Source: CAD feature listing. Evaluate the final solid. Frame: model axes, mm. A direction names the side the tool comes from. Coordinates: 2 decimals unless noted, no trailing zeros. Order: outer loops, then holes, each group sorted by start corner. A loop starts at its lowest first (then second) coordinate and runs counter-clockwise, first axis right, second up.
Item 1: Section A-A on x = 9. Return the cut outline in (y, z).
Item 2: Contact query for flat-ended pins moving along their axis: P1, Ø7.5, axis at x = -8, y = -24, coming from the -Z side; P2, Ø12, axis at y = -14.5, z = 5.5, coming from the +X side; P3, Ø1, axis at x = 31, z = 12, coming from the +Y side; P4, Ø5, axis at x = 9, y = -7, coming from the -Z side. Output: stop coordinate, or through.
Item 3: Section C-C on y = 3. Return the cut outline in (x, z), then the cut area to 3 significant figures.
Item 4: Section D-D on z = 13.5. Return the cut outline in (x, y), then the cut area to 3 significant figures.
Item 5: Section B-B on z = 2.25. Return the cut outline in (x, y), then the cut area to 3 significant figures.
Item 6: Mould query, pull axis Y, two halves, no side actions, for faces 1 (the cylindrical face through (8.404, -9.685, 9.86)), 2 (the flat face through (0, 8, 10)), 3 (the flat face through (-7.804, 7.534, 9.86)), 4 (the cylindrical face through (-2.038, -28.315, 14.93)). Classes: released by +Y, released by -Y, zero draft, split by the parting line, or undercut.
Item 7: Ray query, line 1 (Y direction, x = 9, z = 4.5); line 2 (X direction, y = 5.5, z = 1.25); line 3 (X direction, y = 6, z = 16.5). Return the intervals inside material, ascending.
Item 8: Reachability of faces 5 (the flat face through (32.644, -13.92, 9.86)), 6 (the flat face through (24, 13.085, 10)), 7 (the flat face through (17.5, 7, 10)) from +Z, -Z, +X, -X, +Y, -Y: full face, straight path, thin tool, end or side. Return the list, or none.
from build123d import *
from OCP.BRepFilletAPI import BRepFilletAPI_MakeChamfer

# Parameters (mm, degrees)
SKETCH_1_R          = 2.75
EXTRUDE_1_DEPTH     = 20
CHAMFER_1_SIZE      = 1
CHAMFER_1_SIZE2     = 1.414213562
FILLET_1_R          = 2.5
SKETCH_2_W          = 28.23976686
SKETCH_2_H          = 12.215936495
CUT_EXTRUDE_1_DEPTH = 57.915812899
EXTRUDE_START       = -10
EXTRUDE_2_DEPTH     = 10
SKETCH_4_R          = 1.65
CUT_EXTRUDE_2_DEPTH = 10


with BuildPart() as part:
    # 草图1 → 凸台-拉伸1 (new body)
    with BuildSketch(Plane.XY):
        with BuildLine():
            Line((0, 0), (0, 18))
            Line((0, 18), (-5, 18))
            Line((-5, 18), (-10.312177826, -1.825317547))
            ThreePointArc((-10.312177826, -1.825317547), (-2.044709461, -23.66589163), (21.291049633, -22.769199403))
            Line((21.291049633, -22.769199403), (44.319805153, -4.819805153))
            Line((44.319805153, -4.819805153), (49.319805153, -4.819805153))
            Line((49.319805153, -4.819805153), (17.5, 27))
            Line((17.5, 27), (17.5, 0))
            Line((17.5, 0), (0, 0))
        make_face()
        with Locations((9, -7)):
            Circle(SKETCH_1_R, mode=Mode.SUBTRACT)
    extrude(amount=EXTRUDE_1_DEPTH)

    # 倒角1: one chamfer whose edges measure the first distance from different faces: ONE call of the kernel's chamfer builder (chamfer() names one face for all edges)
    chamfer_1_edges_1 = [part.edges().sort_by_distance(p)[0] for p in [
        (-5, 18, 10),
    ]]
    chamfer_1_side_1 = [part.faces().sort_by_distance(p)[0] for p in [
        (-2.5, 18, 10),
    ]]
    chamfer_1_edges_2 = [part.edges().sort_by_distance(p)[0] for p in [
        (0, 18, 10),
    ]]
    chamfer_1 = BRepFilletAPI_MakeChamfer(part.part.solid().wrapped)
    for e in chamfer_1_edges_1:
        chamfer_1.Add(CHAMFER_1_SIZE, CHAMFER_1_SIZE2, e.wrapped, chamfer_1_side_1[0].wrapped)  # the first distance lies on this face
    for e in chamfer_1_edges_2:
        chamfer_1.Add(CHAMFER_1_SIZE, e.wrapped)
    add(Compound.cast(chamfer_1.Shape()), mode=Mode.REPLACE)

    # 圆角1
    # the kernel refuses this fillet: 2.5 mm, written as the material it takes off along each edge
    with BuildSketch(Plane(origin=(17.5, 27, -15.088834765), x_dir=(0, -1, 0), z_dir=(0, 0, 1))) as fillet_1_piece_1:
        with BuildLine():
            CenterArc((FILLET_1_R * 2.41421356237, FILLET_1_R), FILLET_1_R, 135, 135)
            Line((FILLET_1_R * 1.70710678119, FILLET_1_R * 1.70710678119), (FILLET_1_R * 1.69296464556, FILLET_1_R * 1.72124891681))
            Line((FILLET_1_R * 1.69296464556, FILLET_1_R * 1.72124891681), (-FILLET_1_R * 0.0141421356237, FILLET_1_R * 0.0141421356237))
            Line((-FILLET_1_R * 0.0141421356237, FILLET_1_R * 0.0141421356237), (0, -FILLET_1_R * 0.02))
            Line((0, -FILLET_1_R * 0.02), (FILLET_1_R * 2.41421356237, -FILLET_1_R * 0.02))
            Line((FILLET_1_R * 2.41421356237, -FILLET_1_R * 0.02), (FILLET_1_R * 2.41421356237, 0))
        make_face()
    extrude(amount=50.17766953, mode=Mode.SUBTRACT)
    with BuildSketch(Plane(origin=(49.319805153, -4.819805153, -14.527458022), x_dir=(-0.7071067811865513, 0.7071067811865437, 0), z_dir=(0, 0, 1))) as fillet_1_piece_2:
        with BuildLine():
            CenterArc((5.810983209, 2.5), FILLET_1_R, 155.530199479, 114.469800521)
            Line((3.535533906, 3.535533906), (3.49002492, 3.556244584))
            ThreePointArc((3.49002492, 3.556244584), (1.732411614, 1.803122292), (-0.035355339, 0.035355339))
            Line((-0.035355339, 0.035355339), (0, -0.05))
            Line((0, -0.05), (5.810983209, -0.05))
            Line((5.810983209, -0.05), (5.810983209, 0))
        make_face()
    extrude(amount=49.054916044, mode=Mode.SUBTRACT)

    # 草图2 → 切除-拉伸1 (cut, through all)
    with BuildSketch(Plane.XY.offset(20)):
        with Locations((31.61988343, 19.192534099)):
            Rectangle(SKETCH_2_W, SKETCH_2_H)
    extrude(amount=-CUT_EXTRUDE_1_DEPTH, mode=Mode.SUBTRACT)

    # 草图3 → 凸台-拉伸2 (add)
    with BuildSketch(Plane.XY.offset(20).offset(EXTRUDE_START)):
        with BuildLine():
            ThreePointArc((21.291049633, -22.769199403), (-0.684147296, -24.491564883), (-10.888388441, -4.953159484))
            Line((-10.888388441, -4.953159484), (-13.142676364, -17.190102226))
            ThreePointArc((-13.142676364, -17.190102226), (-6.344046, -32.349558271), (10.241880352, -31.381297238))
            Line((10.241880352, -31.381297238), (21.291049633, -22.769199403))
        make_face()
    extrude(amount=EXTRUDE_2_DEPTH)

    # 草图4 → 切除-拉伸2 (cut)
    with BuildSketch(Plane(origin=(0, 0, 10), x_dir=(-1, 0, 0), z_dir=(0, 0, -1))):
        with Locations((2.25305307, -29.950852035)):
            Circle(SKETCH_4_R)
        with BuildLine():
            Line((-1.24694693, -34.472712807), (-1.24694693, -25.428991263))
            ThreePointArc((-1.24694693, -25.428991263), (-11.630014522, -26.819701675), (-21.291049633, -22.769199403))
            Line((-21.291049633, -22.769199403), (-10.241880352, -31.381297238))
            ThreePointArc((-10.241880352, -31.381297238), (-6.002619266, -33.678292696), (-1.24694693, -34.472712807))
        make_face()
    extrude(amount=-CUT_EXTRUDE_2_DEPTH, mode=Mode.SUBTRACT)


solid = part.part
Answer list:
1. outline: (-26.99, 0) - (-9.75, 0) - (-9.75, 20) - (-26.99, 20) - close; (-4.25, 0) - (0, 0) - (0, 20) - (-4.25, 20) - close
2. P1: stops at z = 10
2. P2: stops at x = 39.6
2. P3: stops at y = 13.08
2. P4: passes through
3. outline: (-9.02, 0) - (0, 0) - (0, 20) - (-9.02, 20) - close; (17.5, 0) - (41.5, 0) - (41.5, 20) - (17.5, 20) - close
3. area: 660 mm2
4. outline: (-13.14, -17.19) arc R14.63 ccw to (1.25, -34.47) - (1.25, -25.43) arc R19.99 ccw to (21.29, -22.77) - (44.32, -4.82) arc R2.5 ccw to (45.21, -0.71) - (31.42, 13.08) - (17.5, 13.08) - (17.5, 0) - (0, 0) - (0, 17) - (-1, 18) - (-4, 18) - (-5.37, 16.63) - (-10.31, -1.83) arc R19.99 ccw to (-10.89, -4.95) - close; hole circle Ø3.3 at (-2.25, -29.95); hole circle Ø5.5 at (9, -7)
4. area: 1,640 mm2
5. outline: (-10.31, -1.83) arc R19.99 ccw to (21.29, -22.77) - (44.32, -4.82) arc R2.5 ccw to (45.21, -0.71) - (31.42, 13.08) - (17.5, 13.08) - (17.5, 0) - (0, 0) - (0, 17) - (-1, 18) - (-4, 18) - (-5.37, 16.63) - close; hole circle Ø5.5 at (9, -7)
5. area: 1,470 mm2
6. face 1: undercut
6. face 2: zero draft
6. face 3: released by +Y
6. face 4: undercut
7. line 1: y = -26.99 to -9.75, -4.25 to 0
7. line 2: x = -8.35 to 0, 17.5 to 39
7. line 3: x = -8.22 to 0, 17.5 to 38.5
8. face 5: +Z, -Z, +X, -Y
8. face 6: +Z, -Z, +X, +Y
8. face 7: +Z, -Z, +Y
